Build history of the part. All positions in model axes, mm. Face numbers are marked on the shaded views. A direction names the side the tool comes from. Give positions to 0.01 mm unless a question says otherwise; leave off trailing zeros. Order: outer loops, then holes, each group sorted by start corner. A loop starts at its lowest first (then second) coordinate and runs counter-clockwise, first axis right, second up. Notation, with made-up numbers: M 54.5,-8.75 L 94.5,-8.75 A24 ccw 94.5,29.25 Z; hole C 41,49.5 d1. An arc over 180 degrees is marked long. Use CSV: the item, a comma, the result in double quotes. Start each with the question number.
Item 1: Band-saw the part on D-D on y = 45. Write the cut outline in (x, z).
Item 2: Two-plate mould, pull along X, no slides. Class the marked faces 4, 5 and 6: pulls with the +X half, pulls with the -X half, needs draft (parallel to the pull), parting line crosses it, or undercut.
Item 3: Band-saw the part on A-A on x = -3.5. Write the cut outline in (y, z), plus the area to 3 significant figures.
Item 4: Which spindle directions (+Z, -Z, +X, -X, +Y, -Y) get a long thin tool onto all of the face, cutting with end or side? Do the marked faces 1, 2 and 3. Say none if no direction does.
Item 5: Band-saw the part on C-C on y = 27. Write the cut outline in (x, z), plus the area to 3 significant figures.
Item 6: Band-saw the part on B-B on z = -0.5. Write the cut outline in (x, y).
Item 7: Wall check: line 1 along Z through (x, y) = (-9, 21.5); line 2 along Z through (x, y) = (-3.5, 14); line 3 along X through (y, z) = (14, 0). Give the ranges that are in metal, low to high.
Item 8: Pin check, flat tips, straight feed: P1, Ø10.5, axis at x = -10, z = 6, coming from the +Y side; P2, Ø22.5, axis at x = 33, y = 41, coming from the +Z side; P3, Ø3, axis at y = 31, z = -6, coming from the -X side; P4, Ø17.5, axis at x = 9, y = 8, coming from the +Z side. Stop position of each tip, or through.
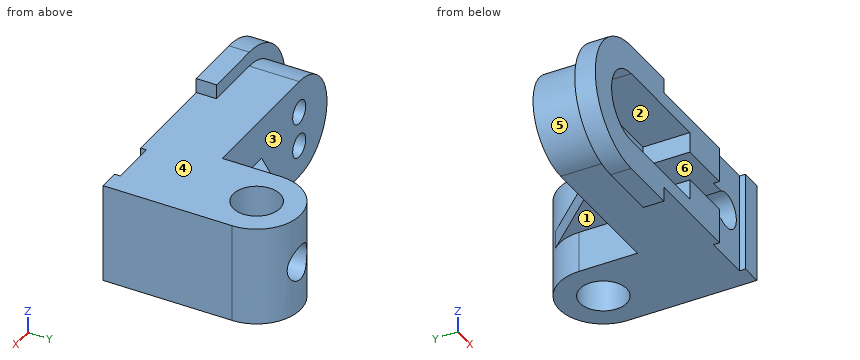
from build123d import *

# Parameters (mm, degrees)
EXTRUDE_1_DEPTH      = 7
EXTRUDE_2_DEPTH      = 17
EXTRUDE_2_DEPTH_BACK = 7
CUT_EXTRUDE_1_DEPTH  = 16
CUT_EXTRUDE_2_REACH  = 76.492
SKETCH_5_R           = 4
SKETCH_6_W           = 30
SKETCH_6_H           = 34
EXTRUDE_3_DEPTH      = 20
EXTRUDE_4_DEPTH      = 34
CUT_EXTRUDE_3_REACH  = 99.422
SKETCH_8_R           = 8
RIB_1_REACH          = 93.946
SKETCH_9_WALL_W      = 227.073790214
SKETCH_9_WALL_H      = 6
SKETCH_10_R          = 6
CUT_EXTRUDE_4_DEPTH  = 92.945634825
SKETCH_11_W          = 16
SKETCH_11_H          = 4
CUT_EXTRUDE_5_DEPTH  = 98.421762397
SKETCH_12_W          = 48.790865184
SKETCH_12_H          = 10
CUT_EXTRUDE_8_DEPTH  = 16


with BuildPart() as part:
    # 草图1 → 凸台-拉伸1 (new body)
    with BuildSketch(Plane(origin=(0, 0, 0), x_dir=(1, 0, 0), z_dir=(0, 1, 0))):
        with BuildLine():
            Line((10, -22), (-10, -22))
            ThreePointArc((-10, -22), (-32, 0), (-10, 22))
            Line((-10, 22), (10, 22))
            Line((10, 22), (10, -22))
        make_face()
    extrude(amount=EXTRUDE_1_DEPTH)

    # 草图3 → 凸台-拉伸2 (add, two sides: drawn at the far end of the back side and taken through both)
    with BuildSketch(Plane(origin=(0, 7, 0), x_dir=(1, 0, 0), z_dir=(0, 1, 0)).offset(-EXTRUDE_2_DEPTH_BACK)):
        with BuildLine():
            Line((-10, 17), (66.999998234, 17))
            Line((66.999998234, 17), (66.999998234, -17))
            Line((66.999998234, -17), (-10.000001766, -17))
            ThreePointArc((-10.000001766, -17), (-27, 8.83e-07), (-10, 17))
        make_face()
    extrude(amount=EXTRUDE_2_DEPTH + EXTRUDE_2_DEPTH_BACK)

    # 草图4 → 切除-拉伸1 (cut)
    with BuildSketch(Plane.XZ):
        with BuildLine():
            Line((-10, 12), (26, 12))
            Line((26, 12), (26, -12))
            Line((26, -12), (-10, -12))
            ThreePointArc((-10, -12), (-22, 0), (-10, 12))
        make_face()
    extrude(amount=-CUT_EXTRUDE_1_DEPTH, mode=Mode.SUBTRACT)

    # 草图5 → 切除-拉伸2 (cut, up to next)
    with BuildSketch(Plane(origin=(0, 24, 0), x_dir=(1, 0, 0), z_dir=(0, 1, 0)), mode=Mode.PRIVATE) as cut_extrude_2_sk1:
        with Locations(Location((-10, 6, 0), (0, 0, 270))):
            Circle(SKETCH_5_R)
    cut_extrude_2_tool1 = extrude(cut_extrude_2_sk1.sketch, amount=-CUT_EXTRUDE_2_REACH, mode=Mode.PRIVATE) & part.part
    # 草图5 → 切除-拉伸2 (cut, up to next)
    with BuildSketch(Plane(origin=(0, 24, 0), x_dir=(1, 0, 0), z_dir=(0, 1, 0)), mode=Mode.PRIVATE) as cut_extrude_2_sk2:
        with Locations(Location((-10, -6, 0), (0, 0, 270))):
            Circle(SKETCH_5_R)
    cut_extrude_2_tool2 = extrude(cut_extrude_2_sk2.sketch, amount=-CUT_EXTRUDE_2_REACH, mode=Mode.PRIVATE) & part.part
    add(cut_extrude_2_tool1.solids().sort_by_distance((-10, 24, -6))[0], mode=Mode.SUBTRACT)
    add(cut_extrude_2_tool2.solids().sort_by_distance((-10, 24, 6))[0], mode=Mode.SUBTRACT)

    # 草图6 → 凸台-拉伸3 (add)
    with BuildSketch(Plane(origin=(0, 24, 0), x_dir=(1, 0, 0), z_dir=(0, 1, 0))):
        with Locations((51.999998234, 0)):
            Rectangle(SKETCH_6_W, SKETCH_6_H)
    extrude(amount=EXTRUDE_3_DEPTH)

    # 草图7 → 凸台-拉伸4 (add)
    with BuildSketch(Plane.XY.offset(17)):
        with BuildLine():
            ThreePointArc((36.999998234, 44), (51.999998234, 59), (66.999998234, 44))
            Line((66.999998234, 44), (36.999998234, 44))
        make_face()
    extrude(amount=-EXTRUDE_4_DEPTH)

    # 草图8 → 切除-拉伸3 (cut, up to next)
    with BuildSketch(Plane.XY.offset(17), mode=Mode.PRIVATE) as cut_extrude_3_sk1:
        with Locations((51.999998234, 44)):
            Circle(SKETCH_8_R)
    cut_extrude_3_tool1 = extrude(cut_extrude_3_sk1.sketch, amount=-CUT_EXTRUDE_3_REACH, mode=Mode.PRIVATE) & part.part
    add(cut_extrude_3_tool1.solids().sort_by_distance((51.999998, 44, 17))[0], mode=Mode.SUBTRACT)

    # 草图9 wall → 筋1 (add, up to next)
    with BuildSketch(Plane(origin=(27.00032198, 39.099368696, 0), x_dir=(0.679915826137, 0.733290167238, 0), z_dir=(-0.733290167238, 0.679915826137, 0)), mode=Mode.PRIVATE) as rib_1_sk1:
        Rectangle(SKETCH_9_WALL_W, SKETCH_9_WALL_H)
    rib_1_tool1 = extrude(rib_1_sk1.sketch, amount=-RIB_1_REACH, mode=Mode.PRIVATE) - part.part
    add(rib_1_tool1.solids().sort_by_distance((27.00032198, 39.099368696, 0))[0])

    # 草图10 → 切除-拉伸4 (cut, through all)
    with BuildSketch(Plane(origin=(0, 59, 0), x_dir=(1, 0, 0), z_dir=(0, 1, 0))):
        with Locations(Location((51.999998234, 0, 0), (0, 0, 270))):
            Circle(SKETCH_10_R)
    extrude(amount=-CUT_EXTRUDE_4_DEPTH, mode=Mode.SUBTRACT)

    # 草图11 → 切除-拉伸5 (cut, through all)
    with BuildSketch(Plane.XY.offset(17)):
        with Locations((51.999998234, 0)):
            Rectangle(SKETCH_11_W, SKETCH_11_H)
    extrude(amount=-CUT_EXTRUDE_5_DEPTH, mode=Mode.SUBTRACT)

    # 草图12 → 切除-拉伸8 (cut)
    with BuildSketch(Plane.XZ):
        with Locations((26, 0)):
            Rectangle(SKETCH_12_W, SKETCH_12_H)
    extrude(amount=-CUT_EXTRUDE_8_DEPTH, mode=Mode.SUBTRACT)


solid = part.part
Model answer:
1,outline,"M 32.47,-3 L 37.03,-3 L 37.03,-17 L 44.06,-17 L 44.06,17 L 37.03,17 L 37.03,3 L 32.47,3 Z; M 59.94,-17 L 66.97,-17 L 66.97,17 L 59.94,17 Z"
2,face 4,"needs draft"
2,face 5,"pulls with the -X half"
2,face 6,"undercut"
3,outline,"M 0,-22 L 7,-22 L 7,-17 L 24,-17 L 24,17 L 7,17 L 7,22 L 0,22 L 0,12 L 16,12 L 16,-12 L 0,-12 Z"
3,area,"502 mm^2"
4,face 1,"-Z, -X, +Y"
4,face 2,"-Y"
4,face 3,"-X, +Y"
5,outline,"M 15.78,-3 L 37,-3 L 37,-17 L 67,-17 L 67,17 L 37,17 L 37,3 L 15.78,3 Z; hole C 52,0 d12"
5,area,"1,030 mm^2"
6,outline,"M -31.99,0 L -21.99,0 L -21.99,16 L 46.02,16 L 46.02,38.68 A8 cw 46.02,49.32 L 46.02,57.76 A15 ccw 41,54.2 L 13,24 L -26.99,24 L -26.99,7 L -31.99,7 Z; M 57.98,2 L 60,2 L 60,0 L 67,0 L 67,44 A15 ccw 57.98,57.76 L 57.98,49.32 A8 cw 57.98,38.68 Z"
7,line 1,"z = -17 to -9.87, -2.13 to 2.13, 9.87 to 17"
7,line 2,"z = -17 to -12, 12 to 17"
7,line 3,"x = -27 to -22, 58 to 67"
8,P1,"stops at y = 24"
8,P2,"stops at z = 17"
8,P3,"stops at x = 37"
8,P4,"stops at z = 22"
